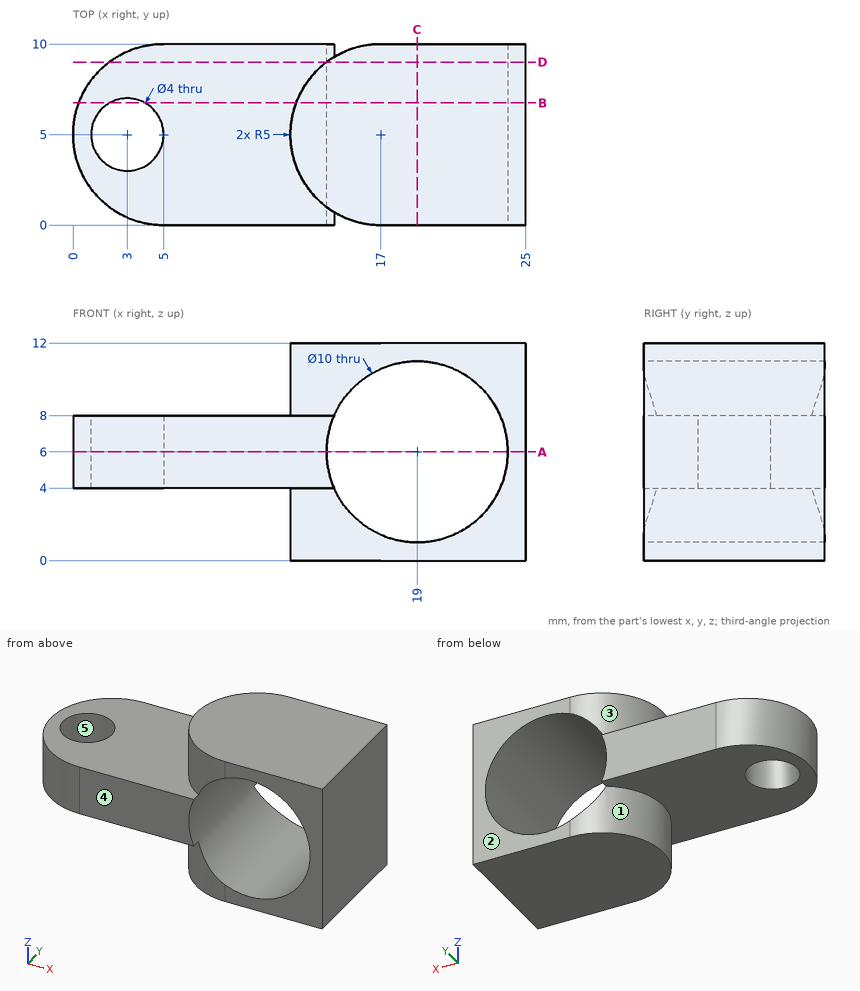
Input: dimensioned drawing with shaded views. Units: mm. Origin: part minimum x, y, z. A direction names the side the tool comes from. Coordinates: 2 decimals unless noted, no trailing zeros. Order: outer loops, then holes, each group sorted by start corner. A loop starts at its lowest first (then second) coordinate and runs counter-clockwise, first axis right, second up.
1. Cut plane C-C, the plane x = 19. Return loops of the section in (y, z).
Checked values:
outline: (0, 0) - (10, 0) - (10, 1) - (0, 1) - close; (0, 11) - (10, 11) - (10, 12) - (0, 12) - close
2. Cut plane A-A, the plane z = 6. Return loops of the section in (x, y), plus the area to 3 significant figures.
Checked values:
outline: (5, 0) - (14, 0) - (14, 10) - (5, 10) arc R5 ccw to start; (24, 0) - (25, 0) - (25, 10) - (24, 10) - close; hole circle Ø4 at (3, 5)
area: 127 mm2
3. Cut plane B-B, the plane y = 6.75. Return loops of the section in (x, z).
Checked values:
outline: (0.32, 4) - (2.03, 4) - (2.03, 8) - (0.32, 8) - close; (3.97, 4) - (12.32, 4) - (12.32, 0) - (25, 0) - (25, 12) - (12.32, 12) - (12.32, 8) - (3.97, 8) - close; hole circle Ø10 at (19, 6)
4. Access query for the marked faces 1 and 2. Directions: +Z, -Z, +X, -X, +Y, -Y. A direction counts if a zero-diameter tool reaches every point of the face in a straight line with its end or side. Return the directions, or none.
Checked values:
face 1: -Z, -X
face 2: +Z, -Z, +X, -X, +Y
5. Cut plane D-D, the plane y = 9. Return loops of the section in (x, z).
Checked values:
outline: (2, 4) - (14, 4) - (14, 0) - (25, 0) - (25, 12) - (14, 12) - (14, 8) - (2, 8) - close; hole circle Ø10 at (19, 6)
6. Draft query along X for the marked faces 3, 4 and 5. Return one class per face: +X half, -X half, draft (parallel to the pull), parting line (faces both ways), or undercut.
Checked values:
face 3: -X half
face 4: draft
face 5: undercut
7. Ray query, line 1 along X through (y, z) = (6, 4.5); line 2 along Z through (x, y) = (14.75, 8.25); line 3 along Z through (x, y) = (19, 4.75). Return the intervals inside material, ascending.
Checked values:
line 1: x = 0.1 to 1.27, 4.73 to 14.23, 23.77 to 25
line 2: z = 0 to 3.37, 8.63 to 12
line 3: z = 0 to 1, 11 to 12
8. Contact query for flat-ended pins moving along their axis: P1, Ø2, axis at y = 3.5, z = 1.5, coming from the -X side; P2, Ø5, axis at x = 3, y = 5, coming from the +Z side. Output: stop coordinate, or through.
Checked values:
P1: stops at x = 12.03
P2: stops at z = 8
